The model under review builds one solid part; all positions refer to its coordinate system, in mm. Face numbers are marked on the shaded views. A direction names the side the tool comes from. Coordinates: 2 decimals unless noted, no trailing zeros. Loops run counter-clockwise (first coordinate to the right, second up) from the corner with the lowest first, then second, coordinate; pieces in that order, holes last. Notation, with made-up numbers: (75.25, 38) - (124.25, 38) arc R27 ccw to (124.25, 61) - close; hole circle Ø8 at (63.5, 49). An arc over 180 degrees is marked (long way). Answer in a Markdown table with one row per item. Add a question column.
(1) Machinability: for the marked faces 5 and 6, which of the approach directions +Z, -Z, +X, -X, +Y, -Y give a long, thin tool a straight path to every point of the face, cutting with its end or side? Answer none if there is none.
(2) For P1, Ø25, axis at x = 43, z = 15.5, coming from the +Y side; P2, Ø5, axis at x = 62.5, y = 8, coming from the +Z side; P3, Ø0.8, axis at x = 66.5, y = 25, coming from the +Z side, all flat-tipped, find the tip position at first contact; note any pin that passes through.
(3) We need section A-A on z = 25. Give the number of separate pieces and of enclosed holes in the cut face, plus the area to 3 significant figures.
(4) We need section B-B on x = 47.95. Write out the cut boundary in (y, z).
(5) For line 1 along X through (y, z) = (-0.8, 25); line 2 along X through (y, z) = (-2.1, 25); line 3 along Z through (x, y) = (64.95, 22) (3 decimals), list the stretches that pass through material, from the lowest coordinate up.
(6) Mouldability with a two-part tool opening along Z and no side actions: class the marked faces 1, 2, 3 and 4 as +Z half, -Z half, draft (parallel to the pull), parting line (faces both ways), or undercut.
(7) We need section D-D on x = 20. Write out the cut boundary in (y, z), plus the area to 3 significant figures.
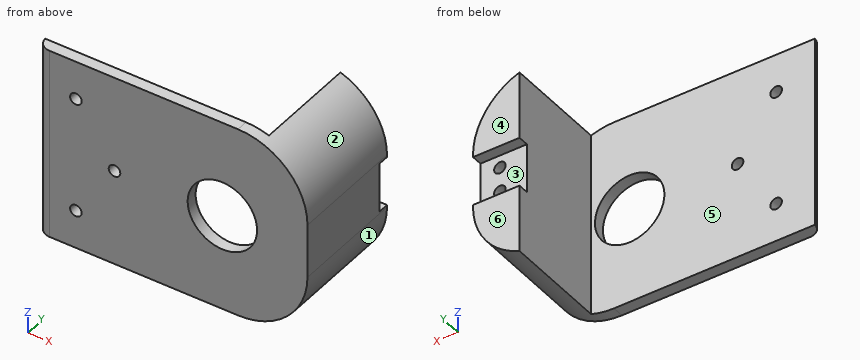
from build123d import *

# Parameters (mm, degrees)
BOSS_EXTRUDE1_DEPTH                        = 50
MOUNTHOLESSKETCH2_R                        = 1.5
MOUNTHOLESSKETCH2_R_2                      = 9
MOUNTHOLESCUT_EXTRUDE1_DEPTH               = 91.160967164
MICROSWITCHCUTSKETCH3_W                    = 12.05
MICROSWITCHCUTSKETCH3_H                    = 12.85
MICROSWITCHCUT_EXTRUDE2_DEPTH              = 2.8
MICROSWITCHMOUNTINGHOLESSKETCH4_R          = 1.5
MICROSWITCHMOUNTINGHOLESCUT_EXTRUDE3_DEPTH = 3
RAILEDGEFILLET1_R                          = 3.125
FRONTEDGEFILLET1_R                         = 18


with BuildPart() as part:
    # ProfileSketch1 → Boss-Extrude1 (new body)
    with BuildSketch(Plane.XY):
        Polygon((70, 0), (70, -3), (0, -3), (0, 0), (57.95, 0), (57.95, 27), (70, 27), align=None)
    extrude(amount=BOSS_EXTRUDE1_DEPTH)

    # MountHolesSketch2 → MountHolesCut-Extrude1 (cut, through all)
    with BuildSketch(Plane(origin=(0, 0, 0), x_dir=(1, 0, 0), z_dir=(0, 1, 0))):
        with Locations(Location((10, -10, 0), (0, 0, 270))):
            Circle(MOUNTHOLESSKETCH2_R)
        with Locations(Location((10, -40, 0), (0, 0, 270))):
            Circle(MOUNTHOLESSKETCH2_R)
        with Locations(Location((47.95, -25, 0), (0, 0, 270))):
            Circle(MOUNTHOLESSKETCH2_R_2)
        with Locations(Location((20, -25, 0), (0, 0, 270))):
            Circle(MOUNTHOLESSKETCH2_R)
    extrude(amount=-MOUNTHOLESCUT_EXTRUDE1_DEPTH, mode=Mode.SUBTRACT)

    # MicroSwitchCutSketch3 → MicroSwitchCut-Extrude2 (cut)
    with BuildSketch(Plane(origin=(0, 27, 0), x_dir=(1, 0, 0), z_dir=(0, 1, 0))):
        with Locations((63.975, -25)):
            Rectangle(MICROSWITCHCUTSKETCH3_W, MICROSWITCHCUTSKETCH3_H)
    extrude(amount=-MICROSWITCHCUT_EXTRUDE2_DEPTH, mode=Mode.SUBTRACT)

    # MicroSwitchMountingHolesSketch4 → MicroSwitchMountingHolesCut-Extrude3 (cut)
    with BuildSketch(Plane(origin=(0, 24.2, 0), x_dir=(1, 0, 0), z_dir=(0, 1, 0))):
        with Locations(Location((64.95, -28.175, 0), (0, 0, 180))):
            Circle(MICROSWITCHMOUNTINGHOLESSKETCH4_R)
        with Locations(Location((64.95, -21.825, 0), (0, 0, 180))):
            Circle(MICROSWITCHMOUNTINGHOLESSKETCH4_R)
    extrude(amount=-MICROSWITCHMOUNTINGHOLESCUT_EXTRUDE3_DEPTH, mode=Mode.SUBTRACT)

    # RailEdgeFillet1
    # the kernel refuses this fillet: 3.125 mm, written as the material it takes off along each edge
    with BuildSketch(Plane(origin=(0, -3, -7.806247498), x_dir=(1, 0, 0), z_dir=(0, 0, 1))) as railedgefillet1_piece_1:
        with BuildLine():
            CenterArc((3.122498999, 3.125), RAILEDGEFILLET1_R, 182.292442776, 87.707557224)
            Line((0, 3), (-0.06244998, 2.9975))
            ThreePointArc((-0.06244998, 2.9975), (-0.0625, 1.5), (-0.0625, 0))
            Line((-0.0625, 0), (0, -0.0625))
            Line((0, -0.0625), (3.122498999, -0.0625))
            Line((3.122498999, -0.0625), (3.122498999, 0))
        make_face()
    extrude(amount=65.612494996, mode=Mode.SUBTRACT)

    # FrontEdgeFillet1
    frontedgefillet1_edges = [part.edges().sort_by_distance(p)[0] for p in [
        (70, 12, 0),
        (70, 12, 50),
    ]]
    fillet(frontedgefillet1_edges, radius=FRONTEDGEFILLET1_R)


solid = part.part
Outcome:
| question | item | result |
|---|---|---|
| 1 | face 5 | +Z, -Z, -X, +Y |
| 1 | face 6 | +Z, -Z, +X, -X, +Y |
| 2 | P1 | y = 0 |
| 2 | P2 | z = 48.12 |
| 2 | P3 | z = 43.19 |
| 3 | separate pieces | 3 |
| 3 | enclosed holes | 0 |
| 3 | area | 437 mm² |
| 4 | outline | (-3, 0) - (0, 0) - (0, 16) - (-3, 16) - close; (-3, 34) - (0, 34) - (0, 50) - (-3, 50) - close |
| 5 | line 1 | 0.14 to 18.5, 21.5 to 38.95, 56.95 to 70 |
| 5 | line 2 | 0.93 to 18.5, 21.5 to 38.95, 56.95 to 70 |
| 5 | line 3 | 5.498 to 20.325, 23.325 to 26.675, 29.675 to 44.502 |
| 6 | face 1 | -Z half |
| 6 | face 2 | +Z half |
| 6 | face 3 | undercut |
| 6 | face 4 | draft |
| 7 | outline | (-3, 0) - (0, 0) - (0, 23.5) - (-3, 23.5) - close; (-3, 26.5) - (0, 26.5) - (0, 50) - (-3, 50) - close |
| 7 | area | 141 mm² |
